Build history of the part. All positions in model axes, mm. Coordinates: 2 decimals unless noted, no trailing zeros. Write each loop counter-clockwise with the first axis right and the second up, starting at its lowest first coordinate (ties: lowest second). Pieces come first, ordered by that corner, then holes.
```python
from build123d import *

# Parameters (mm, degrees)
SKETCH1_R                                    = 32
SKETCH1_R_2                                  = 8.25
BOSS_EXTRUDE1_DEPTH                          = 2
CSK_FOR_M3_HEX_SOCKET_COUNTERSUNK_HE_2_COUNT = 2
CSK_FOR_M3_HEX_SOCKET_COUNTERSUNK_HE_2_PITCH = 11.480502971
CSK_FOR_M3_HEX_SOCKET_COUNTERSUNK_HE_3_COUNT = 2
CSK_FOR_M3_HEX_SOCKET_COUNTERSUNK_HE_3_PITCH = 21.213203436
CSK_FOR_M3_HEX_SOCKET_COUNTERSUNK_HE_4_COUNT = 2
CSK_FOR_M3_HEX_SOCKET_COUNTERSUNK_HE_4_PITCH = 27.716385975
CSK_FOR_M3_HEX_SOCKET_COUNTERSUNK_HE_5_COUNT = 2
CSK_FOR_M3_HEX_SOCKET_COUNTERSUNK_HE_5_PITCH = 30
CSK_FOR_M3_HEX_SOCKET_COUNTERSUNK_HE_6_COUNT = 2
CSK_FOR_M3_HEX_SOCKET_COUNTERSUNK_HE_6_PITCH = 27.716385975
CSK_FOR_M3_HEX_SOCKET_COUNTERSUNK_HE_7_COUNT = 2
CSK_FOR_M3_HEX_SOCKET_COUNTERSUNK_HE_7_PITCH = 21.213203436
CSK_FOR_M3_HEX_SOCKET_COUNTERSUNK_HE_8_COUNT = 2
CSK_FOR_M3_HEX_SOCKET_COUNTERSUNK_HE_8_PITCH = 11.480502971
M3_CLEARANCE_HOLE1_D                         = 3.6


with BuildPart() as part:
    # Sketch1 → Boss-Extrude1 (new body)
    with BuildSketch(Plane(origin=(0, 0, 0), x_dir=(1, 0, 0), z_dir=(0, 1, 0))):
        with Locations(Location((0, 0, 0), (0, 0, 270))):
            Circle(SKETCH1_R)
        with Locations(Location((0, 0, 0), (0, 0, 270))):
            Circle(SKETCH1_R_2, mode=Mode.SUBTRACT)
    extrude(amount=BOSS_EXTRUDE1_DEPTH)

    # Sketch4 → CSK for M3 Hex Socket Countersunk Head Screw1 (revolve, cut)
    with BuildSketch(Plane(origin=(3.882285677, 0, -14.488887394), x_dir=(0, 0, -1), z_dir=(1, 0, 0))):
        Polygon((0, 0), (0, 2), (1.7, 2), (1.7, 1.05), (2.75, 0), align=None)
    csk_for_m3_hex_socket_countersunk_head_s = revolve(axis=Axis((3.882285677, -6.35, -14.488887394), (0, 1, 0)), mode=Mode.SUBTRACT)

    # CSK for M3 Hex Socket Countersunk He 2: CSK for M3 Hex Socket Countersunk Head Screw1 ×2
    with Locations(*[Vector(0.7933533402912735, 0, 0.6087614290086708) * (i * CSK_FOR_M3_HEX_SOCKET_COUNTERSUNK_HE_2_PITCH) for i in range(1, CSK_FOR_M3_HEX_SOCKET_COUNTERSUNK_HE_2_COUNT)]):
        add(csk_for_m3_hex_socket_countersunk_head_s, mode=Mode.SUBTRACT)

    # CSK for M3 Hex Socket Countersunk He 3: CSK for M3 Hex Socket Countersunk Head Screw1 ×2
    with Locations(*[Vector(0.5000000000000544, 0, 0.8660254037844073) * (i * CSK_FOR_M3_HEX_SOCKET_COUNTERSUNK_HE_3_PITCH) for i in range(1, CSK_FOR_M3_HEX_SOCKET_COUNTERSUNK_HE_3_COUNT)]):
        add(csk_for_m3_hex_socket_countersunk_head_s, mode=Mode.SUBTRACT)

    # CSK for M3 Hex Socket Countersunk He 4: CSK for M3 Hex Socket Countersunk Head Screw1 ×2
    with Locations(*[Vector(0.13052619222011386, 0, 0.9914448613738023) * (i * CSK_FOR_M3_HEX_SOCKET_COUNTERSUNK_HE_4_PITCH) for i in range(1, CSK_FOR_M3_HEX_SOCKET_COUNTERSUNK_HE_4_COUNT)]):
        add(csk_for_m3_hex_socket_countersunk_head_s, mode=Mode.SUBTRACT)

    # CSK for M3 Hex Socket Countersunk He 5: CSK for M3 Hex Socket Countersunk Head Screw1 ×2
    with Locations(*[Vector(-0.25881904510246007, 0, 0.9659258262890846) * (i * CSK_FOR_M3_HEX_SOCKET_COUNTERSUNK_HE_5_PITCH) for i in range(1, CSK_FOR_M3_HEX_SOCKET_COUNTERSUNK_HE_5_COUNT)]):
        add(csk_for_m3_hex_socket_countersunk_head_s, mode=Mode.SUBTRACT)

    # CSK for M3 Hex Socket Countersunk He 6: CSK for M3 Hex Socket Countersunk Head Screw1 ×2
    with Locations(*[Vector(-0.6087614290086708, 0, 0.7933533402912735) * (i * CSK_FOR_M3_HEX_SOCKET_COUNTERSUNK_HE_6_PITCH) for i in range(1, CSK_FOR_M3_HEX_SOCKET_COUNTERSUNK_HE_6_COUNT)]):
        add(csk_for_m3_hex_socket_countersunk_head_s, mode=Mode.SUBTRACT)

    # CSK for M3 Hex Socket Countersunk He 7: CSK for M3 Hex Socket Countersunk Head Screw1 ×2
    with Locations(*[Vector(-0.8660254037844073, 0, 0.5000000000000544) * (i * CSK_FOR_M3_HEX_SOCKET_COUNTERSUNK_HE_7_PITCH) for i in range(1, CSK_FOR_M3_HEX_SOCKET_COUNTERSUNK_HE_7_COUNT)]):
        add(csk_for_m3_hex_socket_countersunk_head_s, mode=Mode.SUBTRACT)

    # CSK for M3 Hex Socket Countersunk He 8: CSK for M3 Hex Socket Countersunk Head Screw1 ×2
    with Locations(*[Vector(-0.9914448613738023, 0, 0.13052619222011383) * (i * CSK_FOR_M3_HEX_SOCKET_COUNTERSUNK_HE_8_PITCH) for i in range(1, CSK_FOR_M3_HEX_SOCKET_COUNTERSUNK_HE_8_COUNT)]):
        add(csk_for_m3_hex_socket_countersunk_head_s, mode=Mode.SUBTRACT)

    # M3 Clearance Hole1 (through all)
    with Locations(Plane(origin=(0, 0, 0), x_dir=(-1, 0, 0), z_dir=(0, -1, 0))):
        with Locations((-16.970562748, -16.970562748), (-24, 0), (-16.970562748, 16.970562748), (16.970562748, 16.970562748), (24, 0), (16.970562748, -16.970562748)):
            Hole(M3_CLEARANCE_HOLE1_D / 2)


solid = part.part
```
1. Mould opens along X. For faces 1 (the face through (-31.24, 0.99, -6.94)), 2 (the face through (6.99, 1.52, 11.37)), 3 (the face through (-7, 2, 7)) say: +X half, -X half, draft (parallel to the pull), parting line (faces both ways), or undercut.
Computed values:
face 1: parting line
face 2: undercut
face 3: draft
2. Flat gauge pins, fed straight in: pin 1 (1 mm diameter, centred on y = 1, z = 2.5, fed in from +X); pin 2 (4.5 mm diameter, centred on x = 7.5, z = 12.99, fed in from -Y). Where does each tip first touch, or does it go through?
Computed values:
pin 1: stops at x = 31.94
pin 2: stops at y = 0.5
3. Probe line 1 along Z through (x, y) = (2.5, 1.65); line 2 along X through (y, z) = (0.9, -7); line 3 along X through (y, z) = (1.05, 3). List the from-to ranges inside material, lowest first.
Computed values:
line 1: z = -31.9 to -15.48, -13.5 to -7.86, 7.86 to 31.9
line 2: x = -31.22 to -4.37, 4.37 to 11.21, 14.77 to 31.22
line 3: x = -31.86 to -7.69, 7.69 to 13.04, 15.94 to 31.86
4. Saw through at B-B on x = 0. List the corners of the cut face in (y, z).
Computed values:
outline: (0, -32) - (2, -32) - (2, -8.25) - (0, -8.25) - close; (0, 8.25) - (2, 8.25) - (2, 32) - (0, 32) - close
5. Saw through at A-A on z = 0. List the corners of the cut face in (x, y).
Computed values:
outline: (-32, 0) - (-25.8, 0) - (-25.8, 2) - (-32, 2) - close; (-22.2, 0) - (-8.25, 0) - (-8.25, 2) - (-22.2, 2) - close; (8.25, 0) - (22.2, 0) - (22.2, 2) - (8.25, 2) - close; (25.8, 0) - (32, 0) - (32, 2) - (25.8, 2) - close
6. Saw through at C-C on z = 7.5. List the corners of the cut face in (x, y).
Computed values:
outline: (-31.11, 0) - (-15.74, 0) - (-14.69, 1.05) - (-14.69, 2) - (-31.11, 2) - close; (-11.29, 1.05) - (-10.24, 0) - (-3.44, 0) - (-3.44, 2) - (-11.29, 2) - close; (3.44, 0) - (31.11, 0) - (31.11, 2) - (3.44, 2) - close
7. Saw through at D-D on x = -7.5. List the corners of the cut face in (y, z), plus the area to 3 significant figures.
Computed values:
outline: (0, -31.11) - (2, -31.11) - (2, -14.69) - (1.05, -14.69) - (0, -15.74) - close; (0, -10.24) - (1.05, -11.29) - (2, -11.29) - (2, -3.44) - (0, -3.44) - close; (0, 3.44) - (2, 3.44) - (2, 31.11) - (0, 31.11) - close
area: 103 mm2
